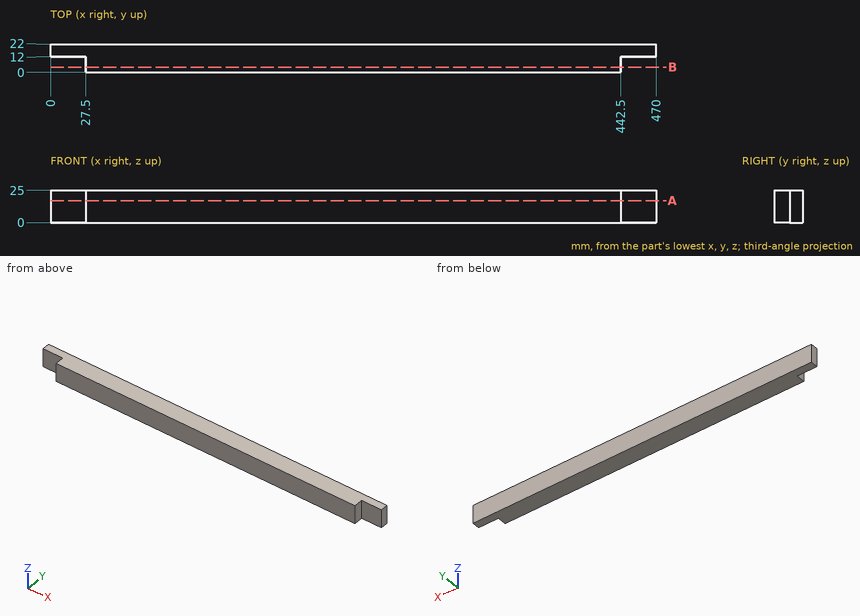
Design review of the part shown in the three views and the two pictorial views. Dimensions are in mm from the part's minimum x, y and z. Round coordinates to 2 decimals unless told otherwise and drop trailing zeros. Loops run counter-clockwise (first coordinate to the right, second up) from the corner with the lowest first, then second, coordinate; pieces in that order, holes last. Notation, with made-up numbers: M 86.25,89 L 129.25,89 A10 cw 129.25,103 Z; hole C 83.25,-23 d8. An arc over 180 degrees is marked long. Write item = value, one per line.
Item 1: Take a section at B-B on y = 4. Write out the cut boundary in (x, z), then the cut area to 3 significant figures.
Return value:
outline = M 27.5,0 L 442.5,0 L 442.5,25 L 27.5,25 Z
area = 10,400 mm2
Item 2: Take a section at A-A on z = 17. Write out the cut boundary in (x, y), then the cut area to 3 significant figures.
Return value:
outline = M 0,12 L 27.5,12 L 27.5,0 L 442.5,0 L 442.5,12 L 470,12 L 470,22 L 0,22 Z
area = 9,680 mm2
Item 3: For line 1 (X direction, y = 10.75, z = 11.5); line 2 (Y direction, x = 451.5, z = 22.25), list the stretches that pass through material, from the lowest coordinate up. Write a range as [from, to].
Return value:
line_1 = [27.5, 442.5]
line_2 = [12, 22]
Item 4: Insertion check: P1, Ø7.5, axis at x = 458, z = 7, coming from the -Y side; P2, Ø6, axis at y = 3.5, z = 20, coming from the -X side; P3, Ø3, axis at y = 8.5, z = 15, coming from the +X side. Each pin has a flat end and moves straight along its axis. Give the tip position at first contact, or say it passes through.
Return value:
P1 = 12
P2 = 27.5
P3 = 442.5
